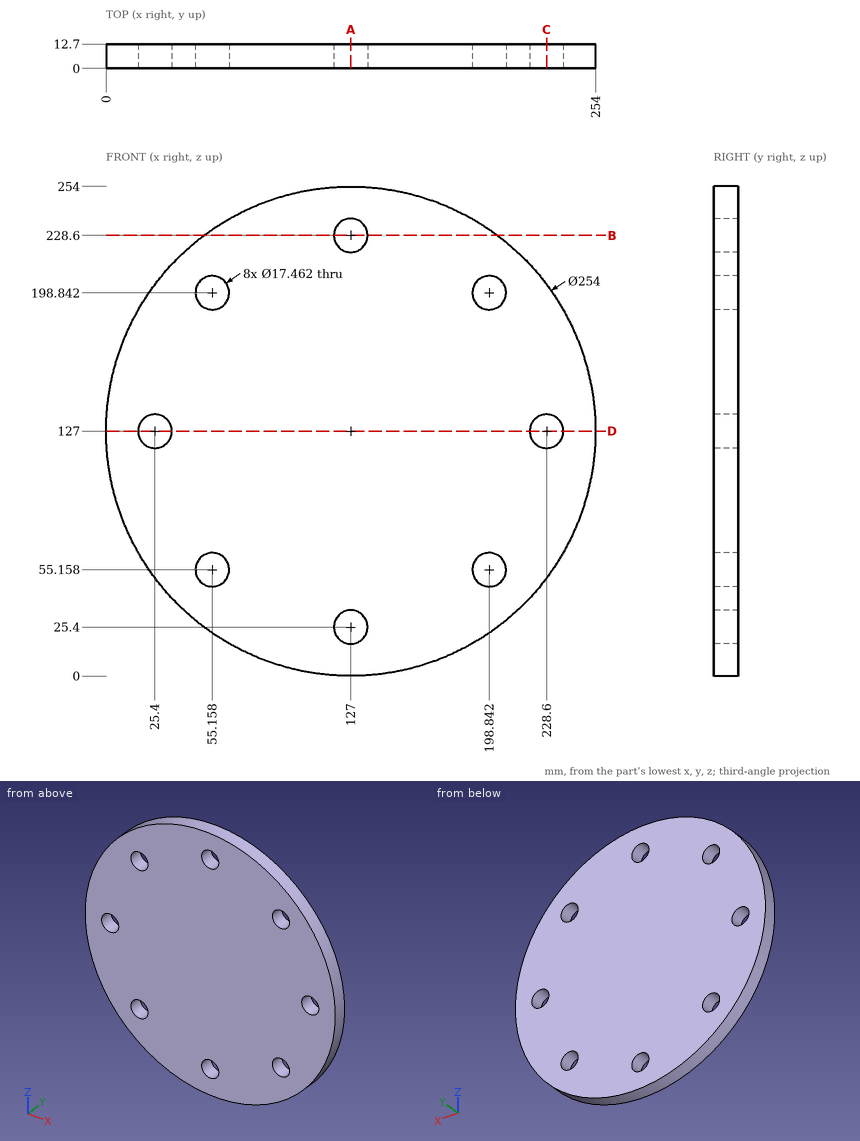
Input: dimensioned drawing with shaded views. Units: mm. Origin: part minimum x, y, z. Coordinates: 2 decimals unless noted, no trailing zeros. Order: outer loops, then holes, each group sorted by start corner. A loop starts at its lowest first (then second) coordinate and runs counter-clockwise, first axis right, second up.
1. Cut plane A-A, the plane x = 127. Return loops of the section in (y, z).
Checked values:
outline: (0, 0) - (12.7, 0) - (12.7, 16.67) - (0, 16.67) - close; (0, 34.13) - (12.7, 34.13) - (12.7, 219.87) - (0, 219.87) - close; (0, 237.33) - (12.7, 237.33) - (12.7, 254) - (0, 254) - close
2. Ray query, line 1 along X through (y, z) = (12, 128) (1 decimal); line 2 along Z through (x, y) = (124.5, 11.75) (1 decimal); line 3 along Z through (x, y) = (197.5, 1) (1 decimal). Return the intervals inside material, ascending.
Checked values:
line 1: x = 0 to 16.7, 34.1 to 219.9, 237.3 to 254
line 2: z = 0 to 17, 33.8 to 220.2, 237 to 254
line 3: z = 21.4 to 46.5, 63.8 to 190.2, 207.5 to 232.6
3. Cut plane B-B, the plane z = 228.6. Return loops of the section in (x, y).
Checked values:
outline: (50.8, 0) - (118.27, 0) - (118.27, 12.7) - (50.8, 12.7) - close; (135.73, 0) - (203.2, 0) - (203.2, 12.7) - (135.73, 12.7) - close
4. Cut plane C-C, the plane x = 228.6. Return loops of the section in (y, z).
Checked values:
outline: (0, 50.8) - (12.7, 50.8) - (12.7, 118.27) - (0, 118.27) - close; (0, 135.73) - (12.7, 135.73) - (12.7, 203.2) - (0, 203.2) - close
5. Contact query for flat-ended pins moving along their axis: P1, Ø22.5, axis at x = 25.4, z = 127, coming from the +Y side; P2, Ø6, axis at x = 68.5, y = 3, coming from the +Z side; P3, Ø6, axis at y = 3, z = 78.5, coming from the +X side; P4, Ø1.5, axis at y = 7, z = 111, coming from the +X side. Output: stop coordinate, or through.
Checked values:
P1: stops at y = 12.7
P2: stops at z = 241.23
P3: stops at x = 245.57
P4: stops at x = 253.08
6. Cut plane D-D, the plane z = 127. Return loops of the section in (x, y), plus the area to 3 significant figures.
Checked values:
outline: (0, 0) - (16.67, 0) - (16.67, 12.7) - (0, 12.7) - close; (34.13, 0) - (219.87, 0) - (219.87, 12.7) - (34.13, 12.7) - close; (237.33, 0) - (254, 0) - (254, 12.7) - (237.33, 12.7) - close
area: 2,780 mm2
